Geometry check sheet. Reference: the model listing, model coordinates, mm. A direction names the side the tool comes from. Round coordinates to 2 decimals unless told otherwise and drop trailing zeros. Order: outer loops, then holes, each group sorted by start corner. A loop starts at its lowest first (then second) coordinate and runs counter-clockwise, first axis right, second up. Notation, with made-up numbers: (55, 30) - (96, 30) arc R29 cw to (96, 66) - close; hole circle Ø11 at (8, -20). An arc over 180 degrees is marked (long way). Write each question's results on one line, items separated by ' | '.
Autodesk Inventor part; units mm, degrees
ref_plane "YZ Plane" through (0, 0, 0) normal (1, 0, 0) x (0, 1, 0)
ref_plane "XZ Plane" through (0, 0, 0) normal (0, 1, 0) x (-1, 0, 0)
ref_plane "XY Plane" through (0, 0, 0) normal (0, 0, 1) x (1, 0, 0)
sketch "Sketch1" plane through (0, 0, 0) normal (0, 0, 1) x (1, 0, 0)
  circle A0 centre (0, 0) radius 50
  line L0 (0, 0) -> (0, 20) construction
  line L1 (2.5, 15) -> (97.5, 15)
  line L2 (97.5, 15) -> (97.5, -15)
  line L3 (97.5, -15) -> (2.5, -15)
  line L4 (2.5, -15) -> (2.5, 15)
  line L5 (2.5, 15) -> (97.5, -15) construction
  line L6 (97.5, 15) -> (2.5, -15) construction
  line L7 (40, 5) -> (60, 5)
  line L8 (60, 5) -> (60, -5)
  line L9 (60, -5) -> (40, -5)
  line L10 (40, -5) -> (40, 5)
  line L11 (40, 5) -> (60, -5) construction
  line L12 (60, 5) -> (40, -5) construction
  line L13 (60, 5) -> (60, 15)
  line L14 (60, -5) -> (60, -15)
  line L15 (-2.5, 15) -> (-97.5, 15)
  line L16 (-97.5, 15) -> (-97.5, -15)
  line L17 (-97.5, -15) -> (-2.5, -15)
  line L18 (-2.5, -15) -> (-2.5, 15)
  line L19 (-2.5, 15) -> (-97.5, -15) construction
  line L20 (-97.5, 15) -> (-2.5, -15) construction
  line L21 (-40, 5) -> (-60, 5)
  line L22 (-60, 5) -> (-60, -5)
  line L23 (-60, -5) -> (-40, -5)
  line L24 (-40, -5) -> (-40, 5)
  line L25 (-40, 5) -> (-60, -5) construction
  line L26 (-60, 5) -> (-40, -5) construction
  line L27 (-60, 5) -> (-60, 15)
  line L28 (-60, -5) -> (-60, -15)
  point P0 (50, 0)
  point P1 (50, 0)
  point P2 (-50, 0)
  point P3 (-50, 0)
  point P4 (49.7494, 5)
  point P5 (49.7494, -5)
  point P6 (-49.7494, -5)
  point P7 (-49.7494, 5)
  dimension "d0" = 100
  dimension "d3" = 20
  dimension "d17" = 95
  dimension "d18" = 30
  dimension "d19" = 20
  dimension "d20" = 10
extrude "Extrusion1" add sketch "Sketch1" along normal blind 5 contours A0 L9 L10 L7 | A0 L7 L8 L9 | L7 L10 L9 A0 L3 L4 L1 | L1 L4 L3 A0 L17 L18 L15 | L13 L1 L2 L3 L14 L8 | L15 L18 L17 A0 L23 L24 L21 | L21 L24 L23 A0 | A0 L23 L22 L21 | L27 L22 L28 L17 L16 L15
sketch "Sketch2" plane through (0, 0, 5) normal (0, 0, 1) x (1, 0, 0)
  line L0 (0, 0) -> (-77.5, 0) construction
  circle A0 centre (-77.5, 0) radius 5.25
  line L1 (0, 0) -> (0, 20) construction
  circle A1 centre (-77.5, 0) radius 8
  circle A2 centre (-69.5, 0) radius 1.75
  circle A3 centre (-77.5, 8) radius 1.75
  circle A4 centre (-85.5, 0) radius 1.75
  circle A5 centre (-77.5, -8) radius 1.75
  circle A6 centre (77.5, 0) radius 5.25
  circle A7 centre (77.5, 0) radius 8
  circle A8 centre (69.5, 0) radius 1.75
  circle A9 centre (77.5, 8) radius 1.75
  circle A10 centre (85.5, 0) radius 1.75
  circle A11 centre (77.5, -8) radius 1.75
  dimension "d26" = 16
  dimension "d6" = 77.5
  dimension "d7" = 10.5
  dimension "d8" = 20
  dimension "d27" = 3.5
  dimension "d30" = 360
extrude "Extrusion2" cut sketch "Sketch2" against normal blind 7 contours A0 | A1 A2 | A1 A2 | A3 A1 | A1 A3 | A5 A1 | A1 A5 | A4 A1 | A1 A4 | A6 | A7 A10 | A7 A10 | A9 A7 | A7 A9 | A11 A7 | A7 A11 | A8 A7 | A7 A8
fillet "Fillet1" radius 3 16 edges at (-60, 5, 2.5) (-60, 15, 2.5) (-49.7494, 5, 2.5) (-60, -5, 2.5) (-60, -15, 2.5) (-49.7494, -5, 2.5) (-97.5, -15, 2.5) (-97.5, 15, 2.5) (97.5, 15, 2.5) (97.5, -15, 2.5) (60, -15, 2.5) (60, 15, 2.5) (60, -5, 2.5) (60, 5, 2.5) (49.7494, 5, 2.5) (49.7494, -5, 2.5)
sketch "Sketch4" plane through (0, 0, 5) normal (0, 0, 1) x (1, 0, 0)
  line L0 (-17.5, 5) -> (17.5, 5)
  line L1 (17.5, 5) -> (17.5, -5)
  line L2 (17.5, -5) -> (-17.5, -5)
  line L3 (-17.5, -5) -> (-17.5, 5)
  line L4 (-17.5, 5) -> (17.5, -5) construction
  line L5 (17.5, 5) -> (-17.5, -5) construction
  circle A0 centre (0, -5) radius 17.5
  circle A1 centre (0, 5) radius 17.5
  circle A2 centre (0, -22.5) radius 4
  circle A3 centre (0, 22.5) radius 4
  circle A4 centre (0, 0) radius 4
  circle A5 centre (16.7705, 0) radius 4
  circle A6 centre (-16.7705, 0) radius 4
  circle A7 centre (0, -12.5) radius 2.5
  circle A8 centre (0, 12.5) radius 2.5
  dimension "d32" = 35
  dimension "d33" = 10
  dimension "d34" = 35
  dimension "d35" = 35
  dimension "d36" = 8
  dimension "d37" = 8
  dimension "d38" = 8
  dimension "d39" = 8
  dimension "d40" = 8
  dimension "d41" = 5
  dimension "d42" = 5
extrude "Extrusion3" cut sketch "Sketch4" against normal blind 10 contours A6 A1 A0 L3 | L3 A6 | A3 A1 | A1 A3 | A6 A0 A1 | A8 A0 | A0 A8 | A6 A1 A0 | A1 A6 A0 | A5 A1 A0 | A0 A1 A5 | A5 L1 | L1 A5 A0 A1 | A0 A5 A1 | A2 A0 | A0 A2 | A7 A1 | A1 A7 | A4
properties part number "TAPA QUE DESPLAZA CON TORNILLOS"
(1) Draft check along Y on faces 1 (the face through (79.169, -7.474, 2.535)), 2 (the face through (97.5, 0, 2)), 3 (the face through (79, -15, 2)), 4 (the face through (82.5, 1.6, 2.5)). Enter one of: released by +Y, released by -Y, zero draft, split by the parting line, or undercut.
Answers follow:
face 1: undercut | face 2: zero draft | face 3: released by -Y | face 4: undercut
(2) Section check C-C (x = 26.5). Record the cut outline in (y, z).
Answers follow:
outline: (-42.4, 0) - (42.4, 0) - (42.4, 5) - (-42.4, 5) - close
(3) Depth check by flat-ended pin: pin 1 Ø2 at (y, z) = (15, 1.5) entering from -X; pin 2 Ø1.5 at (x, z) = (-52.5, 1) entering from +Y; pin 3 Ø1.5 at (x, z) = (-74.5, 1.5) entering from -Y. Enter the tip coordinate at first touch or a pass-through.
Answers follow:
pin 1: x = -96.74 | pin 2: y = 5.07 | pin 3: y = -15
(4) Access from +Z, -Z, +X, -X, +Y, -Y to the whole of each face (thin tool, end or side, straight path). Record for faces 5 (the face through (-79, -15, 2)), 6 (the face through (-60, 10, 2)), 7 (the face through (60, -10, 2)), 8 (the face through (-0.521, 26.466, 2.535)).
Answers follow:
face 5: +Z, -Z, -X, -Y | face 6: +Z, -Z, +Y | face 7: +Z, -Z, -Y | face 8: +Z, -Z
(5) Section check A-A (x = 0). Record the cut outline in (y, z).
Answers follow:
outline: (-50, 0) - (-26.5, 0) - (-26.5, 5) - (-50, 5) - close; (-18.5, 0) - (-15, 0) - (-15, 5) - (-18.5, 5) - close; (-10, 0) - (-4, 0) - (-4, 5) - (-10, 5) - close; (4, 0) - (10, 0) - (10, 5) - (4, 5) - close; (15, 0) - (18.5, 0) - (18.5, 5) - (15, 5) - close; (26.5, 0) - (50, 0) - (50, 5) - (26.5, 5) - close
(6) Section check B-B (y = -22.5). Record the cut outline in (x, z).
Answers follow:
outline: (-44.65, 0) - (-4, 0) - (-4, 5) - (-44.65, 5) - close; (4, 0) - (44.65, 0) - (44.65, 5) - (4, 5) - close
(7) Section check D-D (y = -43.5). Record the cut outline in (x, z), then the cut area to 3 significant figures.
Answers follow:
outline: (-24.65, 0) - (24.65, 0) - (24.65, 5) - (-24.65, 5) - close | area: 247 mm²
(8) Material ranges on line 1 (Y direction, x = 0, z = 0.85); line 2 (Y direction, x = 77.5, z = 3.6); line 3 (X direction, y = 8, z = 3.1), recorded low to high.
Answers follow:
line 1: -50 to -26.5, -18.5 to -15, -10 to -4, 4 to 10, 15 to 18.5, 26.5 to 50 | line 2: -15 to -9.75, -6.25 to -5.25, 5.25 to 6.25, 9.75 to 15 | line 3: -97.5 to -79.25, -75.75 to -60, -49.36 to 49.36, 60 to 75.75, 79.25 to 97.5
